```python
from build123d import *

# Parameters (mm, degrees)
BOSS_EXTRUDE1_DEPTH = 20
FILLET1_R           = 10
SKETCH2_R           = 5
CUT_EXTRUDE1_DEPTH  = 20
SKETCH3_R           = 5
CUT_EXTRUDE2_DEPTH  = 20
SKETCH4_R           = 5
CUT_EXTRUDE3_DEPTH  = 20


with BuildPart() as part:
    # Sketch1 → Boss-Extrude1 (new body)
    with BuildSketch(Plane(origin=(0, 0, 0), x_dir=(0, 0, -1), z_dir=(1, 0, 0))):
        Polygon((0, 0), (479.289321881, 0), (767.012334311, -287.72301243), (802.367673371, -252.367673371), (500, 50), (0, 50), align=None)
    extrude(amount=BOSS_EXTRUDE1_DEPTH)

    # Fillet1
    fillet1_edges = [part.edges().sort_by_distance(p)[0] for p in [
        (10, 0, 0),
        (10, 50, 0),
        (10, 50, -500),
        (10, -252.367673371, -802.367673371),
        (10, -287.72301243, -767.012334311),
        (10, 0, -479.289321881),
    ]]
    fillet(fillet1_edges, radius=FILLET1_R)

    # Sketch2 → Cut-Extrude1 (cut)
    with BuildSketch(Plane(origin=(20, 0, 0), x_dir=(0, 0, -1), z_dir=(1, 0, 0))):
        with Locations((30, 25)):
            Circle(SKETCH2_R)
    extrude(amount=-CUT_EXTRUDE1_DEPTH, mode=Mode.SUBTRACT)

    # Sketch3 → Cut-Extrude2 (cut)
    with BuildSketch(Plane(origin=(20, 0, 0), x_dir=(0, 0, -1), z_dir=(1, 0, 0))):
        with Locations((763.476800406, -248.832139465)):
            Circle(SKETCH3_R)
    extrude(amount=-CUT_EXTRUDE2_DEPTH, mode=Mode.SUBTRACT)

    # Sketch4 → Cut-Extrude3 (cut)
    with BuildSketch(Plane(origin=(20, 0, 0), x_dir=(0, 0, -1), z_dir=(1, 0, 0))):
        with Locations((489.329359641, 24.238795325)):
            Circle(SKETCH4_R)
    extrude(amount=-CUT_EXTRUDE3_DEPTH, mode=Mode.SUBTRACT)


solid = part.part
```
Verification items for the finished model (mm, model axes). A direction names the side the tool comes from. Coordinates: 2 decimals unless noted, no trailing zeros. Write each loop counter-clockwise with the first axis right and the second up, starting at its lowest first coordinate (ties: lowest second). Pieces come first, ordered by that corner, then holes. Notation, with made-up numbers: (-37.5, 9.5) - (12.5, 9.5) arc R31 cw to (12.5, 43.5) - close; hole circle Ø8 at (1.25, -38). An arc over 180 degrees is marked (long way). One line per question, with ' | ' between items. Start each with the question number.
1. Section check C-C (y = -23.5). Enter the section's corners in (x, z), plus the area to 3 significant figures.
2. Section check A-A (x = 3). Enter the section's corners in (y, z).
3. Access from +Z, -Z, +X, -X, +Y, -Y to the whole of each face (thin tool, end or side, straight path). Record for faces 1 (the flat face through (10, -101, -651)), 2 (the flat face through (10, 0, -239)).
4. Material ranges on line 1 along Y through (x, z) = (15.75, -30); line 2 along Y through (x, z) = (8.75, -760.5); line 3 along Y through (x, z) = (5.25, -295.5), recorded low to high.
5. Gauge pin test, flat ends, axial feed: P1, Ø4, axis at x = 9.5, z = -564.5, coming from the +Y side; P2, Ø12, axis at y = -7, z = -454.5, coming from the +X side. Record the tip position at first contact, or that the pin passes through.
6. Section check B-B (z = -94). Enter the section's corners in (x, y).
Computed values:
1) outline: (0, -573.5) - (20, -573.5) - (20, -502.79) - (0, -502.79) - close | area: 1,410 mm²
2) outline: (-280.65, -774.08) - (-259.44, -795.3) arc R10 ccw to (-245.3, -795.3) - (47.07, -502.93) arc R10 ccw to (50, -495.86) - (50, -10) arc R10 ccw to (40, 0) - (10, 0) arc R10 ccw to (0, -10) - (0, -475.15) arc R10 cw to (-2.93, -482.22) - (-280.65, -759.94) arc R10 ccw to start; hole circle Ø10 at (-248.83, -763.48); hole circle Ø10 at (24.24, -489.33); hole circle Ø10 at (25, -30)
3) face 1: -Z, +X, -X, +Y | face 2: +Z, +X, -X, -Y
4) line 1: 0 to 20, 30 to 50 | line 2: -281.17 to -252.85, -244.81 to -210.5 | line 3: 0 to 50
5) P1: y = -12.5 | P2: through
6) outline: (0, 0) - (20, 0) - (20, 50) - (0, 50) - close
